The model under review builds one solid part; all positions refer to its coordinate system, in mm. Face numbers are marked on the shaded views. A direction names the side the tool comes from. Coordinates: 2 decimals unless noted, no trailing zeros. Order: outer loops, then holes, each group sorted by start corner. A loop starts at its lowest first (then second) coordinate and runs counter-clockwise, first axis right, second up. Notation, with made-up numbers: (3, 58.5) -> (8, 58.5) arc R15 cw to (8, 69.5) -> close; hole circle Ø5 at (-32.5, -16). An arc over 180 degrees is marked (long way). Use one line per item in the form item = value. Start each with the question number.
(1) Take a section at B-B (x = 13). State the section outline as (y, z) points.
(2) Wall thickness on line 1 along Y through (x, z) = (13, -1.5); line 2 along Y through (x, z) = (-23, -1.95); line 3 along Z through (x, y) = (6, 14): over which ranges is each line inside the solid? List them lowest first.
(3) For the marked faces 1, 2 and 3, list the 3-axis set-ups (+Z, -Z, +X, -X, +Y, -Y) from which the entire face can be reached by the end or side of a thin tool; tool diameter is ignored.
(4) Take a section at D-D (y = -13). State the section outline as (x, z) points, then the cut area to 3 significant figures.
(5) Take a section at A-A (y = 13). State the section outline as (x, z) points.
(6) Insertion check: pin 1 Ø6 at (x, y) = (12, -4) entering from +Z; pin 2 Ø5 at (x, y) = (1, 5.5) entering from -Z; pin 3 Ø6 at (x, y) = (-9, -14) entering from +Z; pin 4 Ø9.5 at (x, z) = (-1, 6.5) entering from -Y. Each pin has a flat end and moves straight along its axis. Give the tip position at first contact, or say it passes through.
(7) Take a section at C-C (z = 5). State the section outline as (x, y) points, then the cut area to 3 significant figures.
(8) Mouldability with a two-part tool opening along Z and no side actions: class the marked faces 4, 5 and 6 as +Z half, -Z half, draft (parallel to the pull), parting line (faces both ways), or undercut.
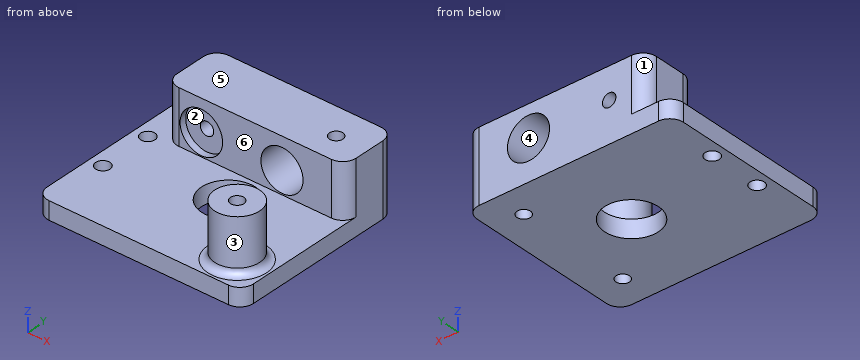
```python
from build123d import *

# Parameters (mm, degrees)
SKETCH_R             = 1.6
SKETCH_R_2           = 6
PAD_DEPTH            = 4
SKETCH001_R          = 5
PAD001_DEPTH         = 12
SKETCH002_R          = 4.7
POCKET_DEPTH         = 13.001
SKETCH003_R          = 4.75
POCKET001_DEPTH      = 1.5
SKETCH004_R          = 1.5
POCKET002_DEPTH      = 13.001
SKETCH005_R          = 1.5
POCKET003_DEPTH      = 4.001
POCKET003_DEPTH_BACK = -12.001
FILLET_R             = 3
FILLET001_R          = 1.5


with BuildPart() as part:
    # Sketch → Pad (new body)
    with BuildSketch(Plane.XY):
        Polygon((0, 20), (-26, 20), (-26, 0), (-26, -20), (0, -20), (20, -20), (20, 0), (20, 20), align=None)
        with Locations((-23, 5.9)):
            Circle(SKETCH_R, mode=Mode.SUBTRACT)
        with Locations((-23, -5.9)):
            Circle(SKETCH_R, mode=Mode.SUBTRACT)
        Circle(SKETCH_R_2, mode=Mode.SUBTRACT)
    extrude(amount=-PAD_DEPTH)

    # Sketch001 → Pad001 (join)
    with BuildSketch(Plane.XY):
        with Locations((13, -13)):
            Circle(SKETCH001_R)
        Polygon((0, 20), (20, 20), (20, 7), (0, 7), (-20, 7), (-20, 20), align=None)
    extrude(amount=PAD001_DEPTH)

    # Sketch002 (on DatumPlane) → Pocket (cut, through all)
    with BuildSketch(Plane.XZ.offset(-7)):
        with Locations((6, 5)):
            Circle(SKETCH002_R)
    extrude(amount=-POCKET_DEPTH, mode=Mode.SUBTRACT)

    # Sketch003 (on DatumPlane) → Pocket001 (cut)
    with BuildSketch(Plane.XZ.offset(-7)):
        with Locations((-12, 5)):
            Circle(SKETCH003_R)
    extrude(amount=-POCKET001_DEPTH, mode=Mode.SUBTRACT)

    # Sketch004 (on DatumPlane) → Pocket002 (cut, through all)
    with BuildSketch(Plane.XZ.offset(-7)):
        with Locations((-12, 5)):
            Circle(SKETCH004_R)
    extrude(amount=-POCKET002_DEPTH, mode=Mode.SUBTRACT)

    # Sketch005 → Pocket003 (cut, two sides)
    with BuildSketch(Plane.XY) as pocket003_sk:
        with Locations((13, -13)):
            Circle(SKETCH005_R)
        with Locations((13, 13)):
            Circle(SKETCH005_R)
    extrude(amount=-POCKET003_DEPTH, mode=Mode.SUBTRACT)
    extrude(pocket003_sk.sketch, amount=-POCKET003_DEPTH_BACK, mode=Mode.SUBTRACT)

    # Fillet
    fillet_edges = [part.edges().sort_by_distance(p)[0] for p in [
        (-26, -20, -2),
        (20, -20, -2),
        (20, 20, -2),
        (-26, 20, -2),
        (20, 7, 6),
        (-20, 7, 6),
        (-20, 20, 6),
    ]]
    fillet(fillet_edges, radius=FILLET_R)

    # Fillet001
    fillet001_edges = [part.edges().sort_by_distance(p)[0] for p in [
        (8, -13, 0),
    ]]
    fillet(fillet001_edges, radius=FILLET001_R)


solid = part.part
```
Findings:
q1.outline = (-20, -4) -> (-14.5, -4) -> (-14.5, 12) -> (-18, 12) -> (-18, 1.5) arc R1.5 cw to (-19.5, 0) -> (-20, 0) -> close; (-11.5, -4) -> (11.5, -4) -> (11.5, 12) -> (7, 12) -> (7, 0) -> (-6.5, 0) arc R1.5 cw to (-8, 1.5) -> (-8, 12) -> (-11.5, 12) -> close; (14.5, -4) -> (20, -4) -> (20, 12) -> (14.5, 12) -> close
q2.line_1 = -20 to -14.5, -11.5 to 11.5, 14.5 to 20
q2.line_2 = -20 to -7.5, -4.3 to 4.3, 7.5 to 20
q2.line_3 = -4 to 0.3, 9.7 to 12
q3.face_1 = +Z, -X, +Y
q3.face_2 = -Y
q3.face_3 = +Z
q4.outline = (-26, -4) -> (11.5, -4) -> (11.5, 12) -> (8, 12) -> (8, 1.5) arc R1.5 cw to (6.5, 0) -> (-26, 0) -> close; (14.5, -4) -> (20, -4) -> (20, 0) -> (19.5, 0) arc R1.5 cw to (18, 1.5) -> (18, 12) -> (14.5, 12) -> close
q4.area = 257 mm²
q5.outline = (-26, -4) -> (11.5, -4) -> (11.5, 12) -> (-20, 12) -> (-20, 0) -> (-26, 0) -> close; (14.5, -4) -> (20, -4) -> (20, 12) -> (14.5, 12) -> close; hole circle Ø3 at (-12, 5); hole circle Ø9.4 at (6, 5)
q6.pin_1 = 0.07
q6.pin_2 = -4
q6.pin_3 = 0
q6.pin_4 = 7
q7.outline = (-20, 10) arc R3 ccw to (-17, 7) -> (-16.75, 7) -> (-16.75, 8.5) -> (-13.5, 8.5) -> (-13.5, 20) -> (-17, 20) arc R3 ccw to (-20, 17) -> close; (-10.5, 8.5) -> (-7.25, 8.5) -> (-7.25, 7) -> (1.3, 7) -> (1.3, 20) -> (-10.5, 20) -> close; circle Ø10 at (13, -13); (10.7, 7) -> (17, 7) arc R3 ccw to (20, 10) -> (20, 17) arc R3 ccw to (17, 20) -> (10.7, 20) -> close; hole circle Ø3 at (13, -13); hole circle Ø3 at (13, 13)
q7.area = 406 mm²
q8.face_4 = undercut
q8.face_5 = +Z half
q8.face_6 = draft
